```python
from build123d import *

# Parameters (mm, degrees)
CHAMFER1_SIZE = 32.258
SCALE1_SCALE  = 0.039370079


with BuildPart() as part:
    # Sketch1 → Revolve1 (revolve)
    with BuildSketch(Plane(origin=(0, 0, 0), x_dir=(0, 0, -1), z_dir=(1, 0, 0))):
        with BuildLine():
            Line((0, 0), (0, 2172.97))
            Line((0, 2172.97), (80.772, 2172.97))
            Line((80.772, 2172.97), (80.772, 456.0493458))
            ThreePointArc((80.772, 456.0493458), (251.373886398, 135.019319557), (612.902, 96.774))
            Line((612.902, 96.774), (677.418, 32.258))
            Line((677.418, 32.258), (677.418, 0))
            Line((677.418, 0), (0, 0))
        make_face()
    revolve(axis=Axis((0, 0, 0), (0, 1, 0)))

    # Chamfer1
    chamfer1_edges = [part.edges().sort_by_distance(p)[0] for p in [
        (0, 2172.97, 80.772),
    ]]
    chamfer(chamfer1_edges, length=CHAMFER1_SIZE)


with BuildPart() as part_1:
    # Scale1: scaled about (0, 313.343453497, 0)
    add(part.part.scale(SCALE1_SCALE).moved(Location((0, 301.00709706, 0))))


solid = part_1.part
```
The listing builds one solid part. Answer for the finished solid, in the listing's coordinates (mm). A direction names the side the tool comes from. Coordinates: 2 decimals unless noted, no trailing zeros. Loops run counter-clockwise (first coordinate to the right, second up) from the corner with the lowest first, then second, coordinate; pieces in that order, holes last. Notation, with made-up numbers: M -10.75,57 L 7.25,57 A27 cw 7.25,83 Z; hole C 76,-9.5 d2. An arc over 180 degrees is marked long. Answer as a JSON object with one key per item and string values. Group by question number.
Item 1: Section C-C (y = 374) is taken. Write down the section's boundary in (x, z).
Item 2: Determine the mould class of faces 3 (the face through (-26.443, 301.633, 3.472)), 4 (the face through (0, 386.557, 0)) for opening direction Z: +Z half, -Z half, draft (parallel to the pull), parting line (faces both ways), or undercut.
Item 3: Which of the six approach directions +Z, -Z, +X, -X, +Y, -Y give full straight-line access (tool end or side, diameter ignored) to faces 1 (the face through (-0.14, 351.66, 3.177)), 2 (the face through (0, 301.007, 0))?
Item 4: Section B-B (x = 0) is taken. Write down the section's boundary in (y, z).
Item 5: Section A-A (z = 0) is taken. Write down the section's boundary in (x, y).
Item 6: Each of these flat-tipped pins is pushed along its axis until it touches: P1, Ø4, axis at x = -20.5, z = 12, coming from the +Y side; P2, Ø3, axis at y = 323.5, z = -2, coming from the +X side; P3, Ø2, axis at y = 376, z = 0.5, coming from the -X side. Where does it stop, or does it pass through?
Item 7: Consider L1, parallel to Y at x = 9, z = -16; L2, parallel to Z at x = 0, y = 328.5; L3, parallel to Y at x = -23, z = 0. Determine where each line is inside the solid, lowest interval first.
Item 8: Section D-D (y = 317) is taken. Write down the section's boundary in (x, z), and give its area (3 significant figures).
Solved:
{
 "1": {"outline": "C 0,0 d6.36"},
 "2": {"face 3": "parting line", "face 4": "draft"},
 "3": {"face 1": "+Y", "face 2": "+Z, -Z, +X, -X, -Y"},
 "4": {"outline": "M 301.01,-26.67 L 302.28,-26.67 L 304.82,-24.13 A15.25 cw 318.96,-3.18 L 385.29,-3.18 L 386.56,-1.91 L 386.56,1.91 L 385.29,3.18 L 318.96,3.18 A15.25 cw 304.82,24.13 L 302.28,26.67 L 301.01,26.67 Z"},
 "5": {"outline": "M -26.67,301.01 L 26.67,301.01 L 26.67,302.28 L 24.13,304.82 A15.25 cw 3.18,318.96 L 3.18,385.29 L 1.91,386.56 L -1.91,386.56 L -3.18,385.29 L -3.18,318.96 A15.25 cw -24.13,304.82 L -26.67,302.28 Z"},
 "6": {"P1": "stops at y = 304.82", "P2": "stops at x = 3.14", "P3": "stops at x = -3.18"},
 "7": {"L1": "y = 301.01 to 303.71", "L2": "z = -3.18 to 3.18", "L3": "y = 301.01 to 304.41"},
 "8": {"outline": "C 0,0 d6.61", "area": "34.4 mm2"}
}
